CAD build for the part. Positions are in the model's coordinates, mm. A direction names the side the tool comes from. Give positions to 0.01 mm unless a question says otherwise; leave off trailing zeros. Loops run counter-clockwise (first coordinate to the right, second up) from the corner with the lowest first, then second, coordinate; pieces in that order, holes last.
```python
from build123d import *

# Parameters (mm, degrees)
POSICIONAMENTOS_R               = 11.1157
BASE_DEPTH                      = 3
FURO_DE_DI_METRO_2_6_2_6_1_D    = 2.6
BASE_DENTE_DEPTH                = 3
RAIO_DENTE_R                    = 1.254921501
PADR_OCIRCULAR1_COUNT           = 10
RAIO_DENTE_OF_PADR_OCIRCULAR1_R = 1.254921501
FURO_DE_DI_METRO_3_0_3_1_D      = 3
ESBO_O9_R                       = 20
CORTE_EXTRUS_O1_DEPTH           = 25.340719016


with BuildPart() as part:
    # Posicionamentos → Base (new body)
    with BuildSketch(Plane.XY):
        Circle(POSICIONAMENTOS_R)
    extrude(amount=BASE_DEPTH)

    # Furo de diâmetro Ø2.6 (2.6)1 (through all)
    with Locations(Plane.XY.offset(3)):
        with Locations((-2.329371406, 8.693332437)):
            Hole(FURO_DE_DI_METRO_2_6_2_6_1_D / 2)

    # Dente → Base Dente (add, through all)
    with BuildSketch(Plane.XY):
        with BuildLine():
            Line((13.415210536, -2.384858144), (10.944111052, -1.945564126))
            ThreePointArc((10.944111052, -1.945564126), (11.1157, 0), (10.944111052, 1.945564126))
            Line((10.944111052, 1.945564126), (13.415210536, 2.384858144))
            ThreePointArc((13.415210536, 2.384858144), (13.875087923, 2.379001106), (14.321480939, 2.268299743))
            ThreePointArc((14.321480939, 2.268299743), (15.956376882, 1.692474606), (17.385445174, 0.711544868))
            ThreePointArc((17.385445174, 0.711544868), (17.4, 0), (17.385445174, -0.711544868))
            ThreePointArc((17.385445174, -0.711544868), (15.956376882, -1.692474606), (14.321480939, -2.268299743))
            ThreePointArc((14.321480939, -2.268299743), (13.875087923, -2.379001106), (13.415210536, -2.384858144))
        make_face()
    base_dente = extrude(amount=BASE_DENTE_DEPTH)

    # Raio Dente
    raio_dente_edges = [part.edges().sort_by_distance(p)[0] for p in [
        (10.944111052, 1.945564126, 1.5),
        (10.944111052, -1.945564126, 1.5),
    ]]
    fillet(raio_dente_edges, radius=RAIO_DENTE_R)

    # PadrãoCircular1: Base Dente ×10 about axis, 5 skipped
    padr_ocircular1_axis = Axis((0, 0, 0), (0, 0, -1))
    add([base_dente.rotate(padr_ocircular1_axis, i * 360 / PADR_OCIRCULAR1_COUNT) for i in range(1, PADR_OCIRCULAR1_COUNT) if i not in (4, 5, 6, 7, 8)])

    # Raio Dente of PadrãoCircular1
    raio_dente_of_padr_ocircular1_edges = [part.edges().sort_by_distance(p)[0] for p in [
        (9.99754573, -4.858792634, 1.5),
        (7.710397929, -8.006781518, 1.5),
        (5.232257744, -9.807255752, 1.5),
        (1.531574863, -11.00968051, 1.5),
        (-1.531574863, -11.00968051, 1.5),
        (-5.232257744, -9.807255752, 1.5),
        (7.710397929, 8.006781518, 1.5),
        (9.99754573, 4.858792634, 1.5),
    ]]
    fillet(raio_dente_of_padr_ocircular1_edges, radius=RAIO_DENTE_OF_PADR_OCIRCULAR1_R)

    # Furo de diâmetro Ø3.0 (3)1 (through all)
    with Locations(Plane.XY.offset(3)):
        with Locations((0, 0)):
            Hole(FURO_DE_DI_METRO_3_0_3_1_D / 2)

    # Esboço9 → Corte-extrusão1 (cut, through all)
    with BuildSketch(Plane.XY):
        with Locations((-24.904867452, -2.178893569)):
            Circle(ESBO_O9_R)
    extrude(amount=CORTE_EXTRUS_O1_DEPTH, mode=Mode.SUBTRACT)


solid = part.part
```
1. Probe line 1 along Y through (x, z) = (0, 0.9); line 2 along X through (y, z) = (-13.5, 1.9); line 3 along X through (y, z) = (9.25, 0.65). List the from-to ranges inside material, lowest first.
Responses:
line 1: y = -11.12 to -1.5, 1.5 to 11.12
line 2: x = -6.62 to -1.88, 1.88 to 6.62
line 3: x = -6.16 to -3.5, -1.15 to 6.16, 8.91 to 14.39
2. Tool access for faces 5 (the face through (-1.785, -12.833, 1.479)), 6 (the face through (-0.446, 11.107, 1.479)), 7 (the face through (13.88, -2.38, 1.48)), 8 (the face through (11.67, 5.67, 1.48)): list every direction of +Z, -Z, +X, -X, +Y, -Y with a clear straight run to the whole face (end or side of a thin tool).
Responses:
face 5: +Z, -Z, -Y
face 6: +Z, -Z, +Y
face 7: +Z, -Z
face 8: +Z, -Z, +X
3. Drop flat-ended pins along their axis: pin 1 (3.5 mm diameter, centred on x = 0, y = 0, fed in from +Z); pin 2 (1 mm diameter, centred on y = -11, z = 2.5, fed in from +X); pin 3 (1 mm diameter, centred on x = 11, z = 1, fed in from -Y). Give the stop position or say it passes through.
Responses:
pin 1: stops at z = 3
pin 2: stops at x = 13.87
pin 3: stops at y = -10.67
4. Saw through at C-C, the plane y = 9.25. List the corners of the cut face in (x, z).
Responses:
outline: (-6.16, 0) - (-3.5, 0) - (-3.5, 3) - (-6.16, 3) - close; (-1.15, 0) - (6.16, 0) - (6.16, 3) - (-1.15, 3) - close; (8.91, 0) - (14.39, 0) - (14.39, 3) - (8.91, 3) - close
5. Saw through at A-A, the plane x = 0. List the corners of the cut face in (y, z), and give its area (3 significant figures).
Responses:
outline: (-11.12, 0) - (-1.5, 0) - (-1.5, 3) - (-11.12, 3) - close; (1.5, 0) - (11.12, 0) - (11.12, 3) - (1.5, 3) - close
area: 57.7 mm2
6. Saw through at B-B, the plane y = 0. List the corners of the cut face in (x, z).
Responses:
outline: (-5.02, 0) - (-1.5, 0) - (-1.5, 3) - (-5.02, 3) - close; (1.5, 0) - (17.4, 0) - (17.4, 3) - (1.5, 3) - close
7. Saw through at D-D, the plane z = 2.1. Count the separate pieces of the cut face and the enclosed holes in it, and give its area (3 significant figures).
Responses:
separate pieces: 1
enclosed holes: 2
area: 429 mm2
8. Pull direction X, two halves, no side cores. Call faces 1 (the face through (6.544, -14.628, 1.479)), 2 (the face through (-2.93, 7.54, 1.48)), 3 (the face through (2, -3, 3)), 4 (the face through (12.78, -2.27, 1.48)): released by +X, released by -X, zero draft, split by the parting line, or undercut.
Responses:
face 1: released by +X
face 2: undercut
face 3: zero draft
face 4: undercut
